CAD build for the part. Positions are in the model's coordinates, mm. A direction names the side the tool comes from. Round coordinates to 2 decimals unless told otherwise and drop trailing zeros. Order: outer loops, then holes, each group sorted by start corner. A loop starts at its lowest first (then second) coordinate and runs counter-clockwise, first axis right, second up. Notation, with made-up numbers: (37.25, 33) - (88.25, 33) arc R29 cw to (88.25, 72) - close; hole circle Ø11 at (-23.75, 9). An arc over 180 degrees is marked (long way). Use one line per item in the form item = value. Start each with the question number.
from build123d import *

# Parameters (mm, degrees)
SKETCH_W     = 6
SKETCH_H     = 40
SKETCH_R     = 1.7
PAD_DEPTH    = 2
FILLET_R     = 2
PAD001_DEPTH = 6
POCKET_DEPTH = 6.001


with BuildPart() as part:
    # Sketch → Pad (new body)
    with BuildSketch(Plane.XY):
        with Locations((0, 17)):
            Rectangle(SKETCH_W, SKETCH_H)
        Circle(SKETCH_R, mode=Mode.SUBTRACT)
        with Locations((0, 34)):
            Circle(SKETCH_R, mode=Mode.SUBTRACT)
    extrude(amount=PAD_DEPTH)

    # Fillet
    fillet_edges = [part.edges().sort_by_distance(p)[0] for p in [
        (-3, -3, 1),
        (-3, 37, 1),
    ]]
    fillet(fillet_edges, radius=FILLET_R)

    # Sketch001 → Pad001 (new body)
    with BuildSketch(Plane.YZ.offset(3)):
        with BuildLine():
            Line((8.669063, 0), (11.110612, 0))
            Line((11.110612, 0), (18.524817, 10.588582))
            ThreePointArc((28.565173, 13.2), (23.064315, 13.742406), (18.524817, 10.588582))
            Line((28.565173, 13.2), (29.436953, 15))
            ThreePointArc((29.436953, 15), (22.560894, 15.678011), (16.886524, 11.735751))
            Line((8.669063, 0), (16.886524, 11.735751))
        make_face()
    extrude(amount=-PAD001_DEPTH)

    # Sketch002 → Pocket (cut, through all)
    with BuildSketch(Plane.YZ.offset(3)):
        Polygon((11.938785, 3.797924), (10.300481, 4.945077), (11.160846, 6.173805), (12.79915, 5.026652), align=None)
        Polygon((13.618302, 4.453075), (12.757937, 3.224347), (13.577089, 2.650771), (14.437454, 3.879499), align=None)
    extrude(amount=-POCKET_DEPTH, mode=Mode.SUBTRACT)


solid = part.part
(1) Slice it at C-C (y = 15). Give the cut face in (x, z), and give its area (3 significant figures).
(2) Flat gauge pins, fed straight in: P1, Ø3, axis at x = 1.5, y = 19.5, coming from the +Z side; P2, Ø1.5, axis at x = 0, y = 11.5, coming from the +Z side; P3, Ø1, axis at x = 0, y = 20, coming from the +Z side; P4, Ø2, axis at x = 0, y = 0, coming from the -Z side. Where does each tip first touch, or does it go through?
(3) Which spindle directions (+Z, -Z, +X, -X, +Y, -Y) get a long thin tool onto all of the face, cutting with end or side? Do faces 1 (the cylindrical face through (-2.43, 36.4, 1.01)), 2 (the cylindrical face through (-0.37, 32.34, 0.99)), 3 (the flat face through (0, 4, 2)), 4 (the flat face through (0.042, 13.194, 3.847)), 5 (the flat face through (0, 25, 2)). Say none if no direction does.
(4) Slice it at D-D (x = -2.5). Give the cut face in (y, z).
(5) Slice it at A-A (y = 0). Give the cut face in (x, z), and give its area (3 significant figures).
(6) Wall check: line 1 (Y direction, x = 0, z = 0.85); line 2 (Z direction, x = -1.5, y = 24); line 3 (Z direction, x = 0.5, y = 28.5). Give the ranges that are in metal, low to high. Write a range as [from, to].
(7) Mould opens along Y. For faces 6 (the cylindrical face through (0.04, 23.14, 13.76)), 7 (the flat face through (1, 37, 1)), 8 (the flat face through (3, 15, 6)), 9 (the flat face through (1, -3, 1)) say: pulls with the +Y half, pulls with the -Y half, needs draft (parallel to the pull), parting line crosses it, or undercut.
(8) Slice it at B-B (x = 0). Give the cut face in (y, z), and give its area (3 significant figures).
Results list:
q1.outline = (-3, 0) - (3, 0) - (3, 2) - (-3, 2) - close; (-3, 5.55) - (3, 5.55) - (3, 9.04) - (-3, 9.04) - close
q1.area = 32.9 mm²
q2.P1 = 15.13
q2.P2 = 4.24
q2.P3 = 14.89
q2.P4 = through
q3.face_1 = +Z, -Z, -X, +Y
q3.face_2 = +Z, -Z
q3.face_3 = +Z, +X, -X, -Y
q3.face_4 = +X, -X
q3.face_5 = +X, -X, +Y
q4.outline = (-2.32, 0) - (36.32, 0) - (36.32, 2) - (12.51, 2) - (13.17, 2.94) - (12.76, 3.22) - (13.62, 4.45) - (14.03, 4.17) - (18.52, 10.59) arc R8 cw to (28.57, 13.2) - (29.44, 15) arc R10 ccw to (16.89, 11.74) - (12.39, 5.31) - (12.8, 5.03) - (11.94, 3.8) - (11.53, 4.08) - (10.07, 2) - (-2.32, 2) - close
q5.outline = (-3, 0) - (-1.7, 0) - (-1.7, 2) - (-3, 2) - close; (1.7, 0) - (3, 0) - (3, 2) - (1.7, 2) - close
q5.area = 5.20 mm²
q6.line_1 = [-3, -1.7], [1.7, 32.3], [35.7, 37]
q6.line_2 = [0, 2], [13.93, 15.94]
q6.line_3 = [0, 2], [13.23, 15.4]
q7.face_6 = undercut
q7.face_7 = pulls with the +Y half
q7.face_8 = needs draft
q7.face_9 = pulls with the -Y half
q8.outline = (-3, 0) - (-1.7, 0) - (-1.7, 2) - (-3, 2) - close; (1.7, 0) - (32.3, 0) - (32.3, 2) - (12.51, 2) - (13.17, 2.94) - (12.76, 3.22) - (13.62, 4.45) - (14.03, 4.17) - (18.52, 10.59) arc R8 cw to (28.57, 13.2) - (29.44, 15) arc R10 ccw to (16.89, 11.74) - (12.39, 5.31) - (12.8, 5.03) - (11.94, 3.8) - (11.53, 4.08) - (10.07, 2) - (1.7, 2) - close; (35.7, 0) - (37, 0) - (37, 2) - (35.7, 2) - close
q8.area = 113 mm²
